Here's how the part is built. I have some questions about the finished solid (model axes, mm). A direction names the side the tool comes from. Coordinates: 2 decimals unless noted, no trailing zeros. Write each loop counter-clockwise with the first axis right and the second up, starting at its lowest first coordinate (ties: lowest second). Pieces come first, ordered by that corner, then holes. Notation, with made-up numbers: (-12.5, 7.25) -> (25.5, 7.25) arc R20 cw to (25.5, 40.25) -> close; hole circle Ø11 at (78.5, 46). An arc over 180 degrees is marked (long way). Answer in a Markdown table with one row per item. Add a question column.
from build123d import *

# Parameters (mm, degrees)
F0_W     = 100
F0_H     = 100
F1_DEPTH = 100
F2_W     = 100
F2_H     = 80
F3_DEPTH = 40
F4_W     = 60
F4_H     = 40
F5_DEPTH = 50.001


with BuildPart() as f1:
    # F0 (on Top) → F1 (new body)
    with BuildSketch(Plane.XY):
        Rectangle(F0_W, F0_H)
    extrude(amount=F1_DEPTH)

    # F2 (on face) → F3 (cut)
    with BuildSketch(Plane.XY.offset(100)):
        with Locations((0, -10)):
            Rectangle(F2_W, F2_H)
    extrude(amount=-F3_DEPTH, mode=Mode.SUBTRACT)

    # F4 (on Front) → F5 (cut, through all)
    with BuildSketch(Plane.XZ):
        with Locations((-21.424717, 0)):
            Rectangle(F4_W, F4_H)
    extrude(amount=-F5_DEPTH, mode=Mode.SUBTRACT)


solid = f1.part
Q1. Imagine slicing it at A-A on x = -30.5. Please give me the cut outline in (y, z), plus the area to 3 significant figures.
Q2. I need wall thicknesses on line 1 (Z direction, x = -3, y = 32.5); line 2 (Z direction, x = -27, y = 5.5); line 3 (Y direction, x = -39.5, z = 85). Which ranges of each line are inside material? Lowest first, please. Write a range as [from, to].
Q3. Imagine slicing it at C-C on y = 11. Please give me the cut outline in (x, z), plus the area to 3 significant figures.
Q4. I'm going to push flat-ended pins straight in: P1, Ø22, axis at x = -23, z = 7.5, coming from the +Y side; P2, Ø20, axis at x = -14, z = 84.5, coming from the -Y side. Where does each tip first touch, or does it pass through?
Q5. Imagine slicing it at B-B on z = 10. Please give me the cut outline in (x, y), plus the area to 3 significant figures.
Q6. Imagine slicing it at D-D on y = -13.5. Please give me the cut outline in (x, z), plus the area to 3 significant figures.
Q7. For faces 1 (the flat face through (-1, 30, 80)), 2 (the flat face through (10, -10, 0)), 3 (the flat face through (-21, 25, 20)), which set-ups out of +Z, -Z, +X, -X, +Y, -Y let a thin tool reach every point of the face, with its end or its side?
Result sheet:
| question | item | result |
|---|---|---|
| 1 | outline | (-50, 0) -> (0, 0) -> (0, 20) -> (50, 20) -> (50, 100) -> (30, 100) -> (30, 60) -> (-50, 60) -> close |
| 1 | area | 5,800 mm^2 |
| 2 | line 1 | z = [20, 100] |
| 2 | line 2 | z = [20, 60] |
| 2 | line 3 | y = [30, 50] |
| 3 | outline | (-50, 20) -> (8.58, 20) -> (8.58, 0) -> (50, 0) -> (50, 60) -> (-50, 60) -> close |
| 3 | area | 4,830 mm^2 |
| 4 | P1 | stops at y = 0 |
| 4 | P2 | stops at y = 30 |
| 5 | outline | (-50, -50) -> (50, -50) -> (50, 50) -> (8.58, 50) -> (8.58, 0) -> (-50, 0) -> close |
| 5 | area | 7,070 mm^2 |
| 6 | outline | (-50, 0) -> (50, 0) -> (50, 60) -> (-50, 60) -> close |
| 6 | area | 6,000 mm^2 |
| 7 | face 1 | +Z, +X, -X, -Y |
| 7 | face 2 | -Z, +X, -X, +Y, -Y |
| 7 | face 3 | -Z, -X, +Y |
